Design review of the part built by this model. Coordinates are the model's own, in mm. A direction names the side the tool comes from. Round coordinates to 2 decimals unless told otherwise and drop trailing zeros. Write each loop counter-clockwise with the first axis right and the second up, starting at its lowest first coordinate (ties: lowest second). Pieces come first, ordered by that corner, then holes. Notation, with made-up numbers: (57, -25) - (110, -25) arc R16 cw to (110, -21) - close; hole circle Ø8 at (81, 17.25). An arc over 180 degrees is marked (long way). Use one line per item in the form item = value.
```python
from build123d import *

# Parameters (mm, degrees)
SKETCH003_W     = 120
SKETCH003_H     = 80
PAD_DEPTH       = 10
SKETCH004_R     = 1.25
POCKET_DEPTH    = 10.001
SKETCH006_R     = 11.05
POCKET002_DEPTH = 10.001
CHAMFER_SIZE    = 3
SKETCH010_R     = 11.015
SKETCH010_R_2   = 1.5
POCKET006_DEPTH = 10.001
SKETCH011_R     = 2.75
POCKET007_DEPTH = 6
SKETCH012_R     = 35.1
POCKET008_DEPTH = 1
POCKET009_DEPTH = 10.001


with BuildPart() as part:
    # Sketch003 → Pad (new body)
    with BuildSketch(Plane.XY):
        Rectangle(SKETCH003_W, SKETCH003_H)
    extrude(amount=-PAD_DEPTH)

    # Sketch004 (on Face5 of Pad) → Pocket (cut, through all)
    with BuildSketch(Plane.XY):
        with Locations((-22.627417, 22.627417)):
            Circle(SKETCH004_R)
        with Locations((0, 32)):
            Circle(SKETCH004_R)
        with Locations((22.627417, 22.627417)):
            Circle(SKETCH004_R)
        with Locations((32, 0)):
            Circle(SKETCH004_R)
        with Locations((22.627417, -22.627417)):
            Circle(SKETCH004_R)
        with Locations((0, -32)):
            Circle(SKETCH004_R)
        with Locations((-22.627417, -22.627417)):
            Circle(SKETCH004_R)
        with Locations((-32, 0)):
            Circle(SKETCH004_R)
    extrude(amount=-POCKET_DEPTH, mode=Mode.SUBTRACT)

    # Sketch006 → Pocket002 (cut, through all)
    with BuildSketch(Plane.XY):
        Circle(SKETCH006_R)
    extrude(amount=-POCKET002_DEPTH, mode=Mode.SUBTRACT)

    # Chamfer
    chamfer_edges = [part.edges().sort_by_distance(p)[0] for p in [
        (60, -40, -5),
        (60, 40, -5),
        (-60, 40, -5),
        (-60, -40, -5),
    ]]
    chamfer(chamfer_edges, length=CHAMFER_SIZE)

    # Sketch010 (on Face5 of Pad) → Pocket006 (cut, through all)
    with BuildSketch(Plane.XY):
        Circle(SKETCH010_R)
        with Locations((-15.5, 15.5)):
            Circle(SKETCH010_R_2)
        with Locations((15.5, 15.5)):
            Circle(SKETCH010_R_2)
        with Locations((15.5, -15.5)):
            Circle(SKETCH010_R_2)
        with Locations((-15.5, -15.5)):
            Circle(SKETCH010_R_2)
    extrude(amount=-POCKET006_DEPTH, mode=Mode.SUBTRACT)

    # Sketch011 (on Face4 of Pocket) → Pocket007 (cut)
    with BuildSketch(Plane.XY):
        with Locations((-29.564145, -12.24587)):
            Circle(SKETCH011_R)
        with Locations((29.564145, 12.24587)):
            Circle(SKETCH011_R)
    extrude(amount=-POCKET007_DEPTH, mode=Mode.SUBTRACT)

    # Sketch012 (on Face4 of Pocket002) → Pocket008 (cut)
    with BuildSketch(Plane.XY):
        Circle(SKETCH012_R)
    extrude(amount=-POCKET008_DEPTH, mode=Mode.SUBTRACT)

    # Sketch013 (on Face2 of Pocket008) → Pocket009 (cut, through all)
    with BuildSketch(Plane.XY):
        with BuildLine():
            ThreePointArc((-41.5, 33.25), (-44.75, 30), (-41.5, 26.75))
            Line((-41.5, 26.75), (-38.5, 26.75))
            ThreePointArc((-38.5, 26.75), (-35.25, 30), (-38.5, 33.25))
            Line((-38.5, 33.25), (-41.5, 33.25))
        make_face()
        with BuildLine():
            ThreePointArc((38.5, 33.25), (35.25, 30), (38.5, 26.75))
            Line((38.5, 26.75), (41.5, 26.75))
            ThreePointArc((41.5, 26.75), (44.75, 30), (41.5, 33.25))
            Line((41.5, 33.25), (38.5, 33.25))
        make_face()
        with BuildLine():
            ThreePointArc((-41.5, -26.75), (-44.75, -30), (-41.5, -33.25))
            Line((-41.5, -33.25), (-38.5, -33.25))
            ThreePointArc((-38.5, -33.25), (-35.25, -30), (-38.5, -26.75))
            Line((-38.5, -26.75), (-41.5, -26.75))
        make_face()
        with BuildLine():
            ThreePointArc((38.5, -26.75), (35.25, -30), (38.5, -33.25))
            Line((38.5, -33.25), (41.5, -33.25))
            ThreePointArc((41.5, -33.25), (44.75, -30), (41.5, -26.75))
            Line((41.5, -26.75), (38.5, -26.75))
        make_face()
    extrude(amount=-POCKET009_DEPTH, mode=Mode.SUBTRACT)


solid = part.part
```
Q1. Draft analysis for pull direction X (two halves, no side actions). For faces 4 (the flat face through (59, -38, -5)), 5 (the cylindrical face through (35.25, -29.93, -4.93)), 6 (the flat face through (-14, 1, -10)), state which applies: released by +X, released by -X, zero draft, split by the parting line, or undercut.
Calculated:
face_4 = released by +X
face_5 = undercut
face_6 = zero draft
Q2. We need section A-A on x = 0. Write out the cut boundary in (y, z), then the cut area to 3 significant figures.
Calculated:
outline = (-40, -10) - (-33.25, -10) - (-33.25, -1) - (-35.1, -1) - (-35.1, 0) - (-40, 0) - close; (-30.75, -10) - (-11.05, -10) - (-11.05, -1) - (-30.75, -1) - close; (11.05, -10) - (30.75, -10) - (30.75, -1) - (11.05, -1) - close; (33.25, -10) - (40, -10) - (40, 0) - (35.1, 0) - (35.1, -1) - (33.25, -1) - close
area = 486 mm2
Q3. For P1, Ø21, axis at x = 17, y = 7.5, coming from the +Z side; P2, Ø13.5, axis at x = 0, y = 0, coming from the -Z side, all flat-tipped, find the tip position at first contact; note any pin that passes through.
Calculated:
P1 = -1
P2 = through
Q4. We need section B-B on y = 32. Write out the cut boundary in (x, z), then the cut area to 3 significant figures.
Calculated:
outline = (-60, -10) - (-44.06, -10) - (-44.06, 0) - (-60, 0) - close; (-35.94, -10) - (-1.25, -10) - (-1.25, -1) - (-14.42, -1) - (-14.42, 0) - (-35.94, 0) - close; (1.25, -10) - (35.94, -10) - (35.94, 0) - (14.42, 0) - (14.42, -1) - (1.25, -1) - close; (44.06, -10) - (60, -10) - (60, 0) - (44.06, 0) - close
area = 986 mm2
Q5. To check wall thickness, follow line 1 along Y through (x, z) = (15.5, -5.25); line 2 along Y through (x, z) = (0, -0.3); line 3 along X through (y, z) = (-27, -2.5). State the ranges of each line that lie inside material, in increasing order. Write a range as from..to.
Calculated:
line_1 = -40..-17, -14..14, 17..40
line_2 = -40..-35.1, 35.1..40
line_3 = -60..-42.75, -37.25..37.25, 42.75..60
Q6. Machinability: for faces 1 (the flat face through (-8, 8, -1)), 2 (the flat face through (-1, -40, -5)), 3 (the flat face through (40, -26.75, -5)), which of the approach directions +Z, -Z, +X, -X, +Y, -Y give a long, thin tool a straight path to every point of the face, cutting with its end or side? Answer none if there is none.
Calculated:
face_1 = +Z
face_2 = +Z, -Z, +X, -X, -Y
face_3 = +Z, -Z
Q7. We need section D-D on z = -8.25. State how many separate pieces and enclosed holes the cut face has, then the cut area to 3 significant figures.
Calculated:
separate_pieces = 1
enclosed_holes = 17
area = 8,920 mm2
Q8. We need section C-C on x = -15.5. Write out the cut boundary in (y, z), then the cut area to 3 significant figures.
Calculated:
outline = (-40, -10) - (-17, -10) - (-17, -1) - (-31.49, -1) - (-31.49, 0) - (-40, 0) - close; (-14, -10) - (14, -10) - (14, -1) - (-14, -1) - close; (17, -10) - (40, -10) - (40, 0) - (31.49, 0) - (31.49, -1) - (17, -1) - close
area = 683 mm2
